Geometry: final body of the model. Coordinates: model frame, mm. Coordinates: 2 decimals unless noted, no trailing zeros. Order: outer loops, then holes, each group sorted by start corner. A loop starts at its lowest first (then second) coordinate and runs counter-clockwise, first axis right, second up. Notation, with made-up numbers: M -37.75,79.25 L 18.25,79.25 A17 ccw 18.25,90.25 Z; hole C 24.25,24 d10. An arc over 180 degrees is marked long. Use CSV: the item, a comma, the result in double quotes. Start each with the question number.
1. Material intervals for line 1 (Z direction, x = 37, y = 1.95); line 2 (Z direction, x = 45.5, y = 1.2); line 3 (X direction, y = 0.55, z = -49), sorted ascending.
2. Section query D-D on z = 19. Return the cut outline in (x, y).
3. Section query A-A on z = 47. Return the cut outline in (x, y).
4. First-contact query: P1, Ø2.5, axis at x = -17.94, z = -33.46, coming from the -Y side; P2, Ø1, axis at x = 16.5, y = 0.5, coming from the -Z side. Flat tips, straight axial feed; report the tip coordinate or a pass-through.
5. Section query C-C on y = 1. State how many separate pieces and enclosed holes the cut face has, and give its area (3 significant figures).
6. Section query B-B on x = 36.5. Return the cut outline in (y, z), and give its area (3 significant figures).
Autodesk Inventor part; units mm, degrees
ref_plane "YZ Plane" through (0, 0, 0) normal (1, 0, 0) x (0, 1, 0)
ref_plane "XZ Plane" through (0, 0, 0) normal (0, 1, 0) x (-1, 0, 0)
ref_plane "XY Plane" through (0, 0, 0) normal (0, 0, 1) x (1, 0, 0)
sketch "Sketch1" plane through (0, 0, 0) normal (0, 1, 0) x (-1, 0, 0)
  arc A0 (-53.7401, -31.1127) -> (-31.1127, -53.7401) centre (-42.4264, -42.4264) ccw
  arc A1 (31.1127, -53.7401) -> (53.7401, -31.1127) centre (42.4264, -42.4264) ccw
  arc A2 (53.7401, 31.1127) -> (31.1127, 53.7401) centre (42.4264, 42.4264) ccw
  arc A3 (-31.1127, 53.7401) -> (-53.7401, 31.1127) centre (-42.4264, 42.4264) ccw
  line L0 (-53.7401, 31.1127) -> (-33.9411, 11.3137)
  line L1 (11.3137, -33.9411) -> (31.1127, -53.7401)
  line L2 (-53.7401, -31.1127) -> (-33.9411, -11.3137)
  line L3 (11.3137, 33.9411) -> (31.1127, 53.7401)
  line L4 (-31.1127, 53.7401) -> (-11.3137, 33.9411)
  line L5 (33.9411, -11.3137) -> (53.7401, -31.1127)
  line L6 (-31.1127, -53.7401) -> (-11.3137, -33.9411)
  line L7 (33.9411, 11.3137) -> (53.7401, 31.1127)
  arc A4 (11.3137, -33.9411) -> (-11.3137, -33.9411) centre (0, -45.2548) ccw
  arc A5 (33.9411, 11.3137) -> (33.9411, -11.3137) centre (45.2548, 0) ccw
  arc A6 (-11.3137, 33.9411) -> (11.3137, 33.9411) centre (0, 45.2548) ccw
  arc A7 (-33.9411, -11.3137) -> (-33.9411, 11.3137) centre (-45.2548, 0) ccw
  arc A8 (-53.7401, -31.1127) -> (-31.1127, -53.7401) centre (-42.4264, -42.4264) ccw
  arc A9 (31.1127, -53.7401) -> (53.7401, -31.1127) centre (42.4264, -42.4264) ccw
  arc A10 (53.7401, 31.1127) -> (31.1127, 53.7401) centre (42.4264, 42.4264) ccw
  arc A11 (-31.1127, 53.7401) -> (-53.7401, 31.1127) centre (-42.4264, 42.4264) ccw
  line L8 (-53.7401, 31.1127) -> (-33.9411, 11.3137)
  line L9 (11.3137, -33.9411) -> (31.1127, -53.7401)
  line L10 (-53.7401, -31.1127) -> (-33.9411, -11.3137)
  line L11 (11.3137, 33.9411) -> (31.1127, 53.7401)
  line L12 (-31.1127, 53.7401) -> (-11.3137, 33.9411)
  line L13 (33.9411, -11.3137) -> (53.7401, -31.1127)
  line L14 (-31.1127, -53.7401) -> (-11.3137, -33.9411)
  line L15 (33.9411, 11.3137) -> (53.7401, 31.1127)
  arc A12 (11.3137, -33.9411) -> (-11.3137, -33.9411) centre (0, -45.2548) ccw
  arc A13 (33.9411, 11.3137) -> (33.9411, -11.3137) centre (45.2548, 0) ccw
  arc A14 (-11.3137, 33.9411) -> (11.3137, 33.9411) centre (0, 45.2548) ccw
  arc A15 (-33.9411, -11.3137) -> (-33.9411, 11.3137) centre (-45.2548, 0) ccw
  arc A16 (-53.7401, -31.1127) -> (-31.1127, -53.7401) centre (-42.4264, -42.4264) ccw
  arc A17 (31.1127, -53.7401) -> (53.7401, -31.1127) centre (42.4264, -42.4264) ccw
  arc A18 (53.7401, 31.1127) -> (31.1127, 53.7401) centre (42.4264, 42.4264) ccw
  arc A19 (-31.1127, 53.7401) -> (-53.7401, 31.1127) centre (-42.4264, 42.4264) ccw
  line L16 (-53.7401, 31.1127) -> (-33.9411, 11.3137)
  line L17 (11.3137, -33.9411) -> (31.1127, -53.7401)
  line L18 (-53.7401, -31.1127) -> (-33.9411, -11.3137)
  line L19 (11.3137, 33.9411) -> (31.1127, 53.7401)
  line L20 (-31.1127, 53.7401) -> (-11.3137, 33.9411)
  line L21 (33.9411, -11.3137) -> (53.7401, -31.1127)
  line L22 (-31.1127, -53.7401) -> (-11.3137, -33.9411)
  line L23 (33.9411, 11.3137) -> (53.7401, 31.1127)
  arc A20 (11.3137, -33.9411) -> (-11.3137, -33.9411) centre (0, -45.2548) ccw
  arc A21 (33.9411, 11.3137) -> (33.9411, -11.3137) centre (45.2548, 0) ccw
  arc A22 (-11.3137, 33.9411) -> (11.3137, 33.9411) centre (0, 45.2548) ccw
  arc A23 (-33.9411, -11.3137) -> (-33.9411, 11.3137) centre (-45.2548, 0) ccw
  point P0 (0, 0)
  point P1 (0, 0)
  point P2 (0, 0)
  point P3 (0, 0)
  point P4 (0, 0)
  point P5 (0, 0)
  point P6 (0, 0)
extrude "Extrusion1" add sketch "Sketch1" along normal blind 2
sketch "Sketch3" plane through (0, 2, 0) normal (0, 1, 0) x (1, 0, 0)
  arc A0 (53.7401, 31.1127) -> (31.1127, 53.7401) centre (42.4264, 42.4264) ccw
  circle A1 centre (42.4264, 42.4264) radius 1.5
  arc A2 (-31.1127, 53.7401) -> (-53.7401, 31.1127) centre (-42.4264, 42.4264) ccw
  circle A3 centre (-42.4264, 42.4264) radius 1.5
  arc A4 (-53.7401, -31.1127) -> (-31.1127, -53.7401) centre (-42.4264, -42.4264) ccw
  circle A5 centre (-42.4264, -42.4264) radius 1.5
  arc A6 (31.1127, -53.7401) -> (53.7401, -31.1127) centre (42.4264, -42.4264) ccw
  circle A7 centre (42.4264, -42.4264) radius 1.5
  circle A8 centre (-31.1127, -31.1127) radius 1.5
  circle A9 centre (31.1127, 31.1127) radius 1.5
  circle A10 centre (-29.9941, -23.2724) radius 1.5
  circle A11 centre (-17.9352, 33.4601) radius 1.5
  circle A12 centre (29.9941, 23.2724) radius 1.5
  circle A13 centre (17.9352, -33.4601) radius 1.5
  point P0 (0, 0)
  dimension "d5" = 3
  dimension "d6" = 3
  dimension "d7" = 3
  dimension "d8" = 3
  dimension "d43" = 3
  dimension "d44" = 3
  dimension "d47" = 3
  dimension "d48" = 3
  dimension "d49" = 3
  dimension "d50" = 3
extrude "Extrusion3" cut sketch "Sketch3" against normal blind 20
properties part number "platform 1"
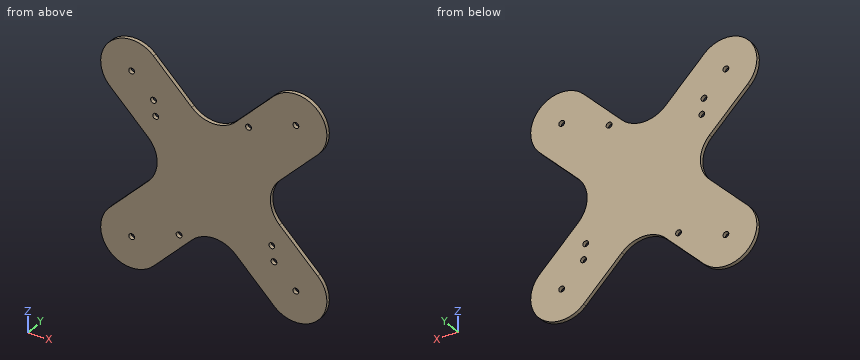
Results list:
1,line 1,"z = -57.48 to -14.37, 14.37 to 57.48"
1,line 2,"z = -58.13 to -22.87, 22.87 to 58.13"
1,line 3,"x = -57.01 to -26.37, 26.37 to 57.01"
2,outline,"M -41.63,0 L 41.63,0 L 41.63,2 L -41.63,2 Z"
3,outline,"M -57.76,0 L -24.37,0 L -24.37,2 L -57.76,2 Z; M 24.37,0 L 57.76,0 L 57.76,2 L 24.37,2 Z"
4,P1,"passes through"
4,P2,"stops at z = -39.63"
5,separate pieces,"1"
5,enclosed holes,"10"
5,area,"8,410 mm²"
6,outline,"M 0,-57.29 L 2,-57.29 L 2,-13.87 L 0,-13.87 Z; M 0,13.87 L 2,13.87 L 2,57.29 L 0,57.29 Z"
6,area,"174 mm²"
